Autodesk Inventor part; units mm, degrees
ref_plane "YZ Plane" through (0, 0, 0) normal (1, 0, 0) x (0, 1, 0)
ref_plane "XZ Plane" through (0, 0, 0) normal (0, 1, 0) x (-1, 0, 0)
ref_plane "XY Plane" through (0, 0, 0) normal (0, 0, 1) x (1, 0, 0)
sketch "Sketch1" plane through (0, 0, 0) normal (0, 0, 1) x (1, 0, 0)
  line L0 (-107.95, 63.5) -> (107.95, 63.5)
  line L1 (107.95, 63.5) -> (107.95, -63.5)
  line L2 (107.95, -63.5) -> (-107.95, -63.5)
  line L3 (-107.95, -63.5) -> (-107.95, 63.5)
  line L4 (-107.95, 63.5) -> (107.95, -63.5) construction
  line L5 (107.95, 63.5) -> (-107.95, -63.5) construction
  point P0 (0, 0)
  dimension "d0" = 215.9
  dimension "d1" = 127
extrude "Extrusion1" add sketch "Sketch1" along normal blind 317.5
fillet "Fillet1" radius 10 12 edges at (0, 63.5, 317.5) (-107.95, 63.5, 158.75) (0, 63.5, 0) (107.95, 63.5, 158.75) (107.95, 0, 317.5) (107.95, -63.5, 158.75) (107.95, 0, 0) (0, -63.5, 317.5) (-107.95, 0, 317.5) (0, -63.5, 0) (-107.95, 0, 0) (-107.95, -63.5, 158.75)
sketch "Sketch4" plane through (-97.95, 63.5, 10) normal (0, 1, 0) x (1, 0, 0)
  line L0 (10, -10) -> (185.9, -10)
  line L1 (185.9, -10) -> (185.9, -287.5)
  line L2 (185.9, -287.5) -> (10, -287.5)
  line L3 (10, -287.5) -> (10, -10)
  line L4 (0, 0) -> (195.9, 0)
  line L5 (195.9, 0) -> (195.9, -297.5)
  line L6 (195.9, -297.5) -> (0, -297.5)
  line L7 (0, -297.5) -> (0, 0)
  point P0 (97.95, 10)
  point P1 (97.95, -10)
  dimension "d20" = 10
  dimension "d21" = 10
  dimension "d22" = 10
  dimension "d23" = 10
extrude "Extrusion4" cut sketch "Sketch4" against normal blind 110 contours L0 L1 L2 L3
sketch "Sketch5" plane through (107.95, -53.5, 10) normal (1, 0, 0) x (0, 0, -1)
  circle A0 centre (-267.75, 94.1117) radius 10
  circle A1 centre (-208.25, 94.1117) radius 10
  circle A2 centre (-148.75, 94.1117) radius 10
  circle A3 centre (-89.25, 94.1117) radius 10
  circle A4 centre (-29.75, 94.1117) radius 10
  line L0 (-297.5, 107) -> (-297.5, 0)
  point P0 (10, 53.5)
  dimension "d26" = 20
  dimension "d27" = 20
  dimension "d28" = 20
  dimension "d29" = 20
  dimension "d30" = 20
  dimension "d31" = 29.75
  dimension "d32" = 59.5
  dimension "d33" = 59.5
  dimension "d34" = 59.5
  dimension "d35" = 59.5
extrude "Extrusion5" cut sketch "Sketch5" against normal blind 59.5
equation "\"d36\" = d33"
Part model, mm, in its own coordinate system. A direction names the side the tool comes from. Coordinates: 2 decimals unless noted, no trailing zeros. Loops run counter-clockwise (first coordinate to the right, second up) from the corner with the lowest first, then second, coordinate; pieces in that order, holes last. Notation, with made-up numbers: (-14, 16.25) - (42, 16.25) arc R24 ccw to (42, 45.25) - close; hole circle Ø4 at (-5, -36). An arc over 180 degrees is marked (long way). Write item = value, one per line. Start each with the question number.
Item 1: Cut at B-B, the plane y = 23. Give the cut face in (x, z).
Item 2: Cut at A-A, the plane z = 277.75. Give the cut face in (x, y).
Item 3: Cut at D-D, the plane z = 200.5. Give the cut face in (x, y), and give its area (3 significant figures).
Item 4: Flat gauge pins, fed straight in: pin 1 Ø3 at (x, y) = (-27.5, 35) entering from -Z; pin 2 Ø2 at (x, z) = (-69, 129.5) entering from +Y. Where does each tip first touch, or does it go through?
Item 5: Mould opens along Z. For faces 1 (the cylindrical face through (98.09, 36.782, 209.013)), 2 (the cylindrical face through (104.94, -0.75, 2.85)), 3 (the cylindrical face through (105.1, -0.75, 314.49)), 4 (the cylindrical face through (105.1, 60.49, 160.83)) say: released by +Z, released by -Z, zero draft, split by the parting line, or undercut.
Item 6: Wall check: L1, parallel to Y at x = 97, z = 158.75; L2, parallel to X at y = 16.5, z = 152; L3, parallel to Z at x = 34.5, y = 14.5. Give the ranges that are in metal, low to high. Write a range as from..to.
Item 7: Cut at C-C, the plane x = 93.5. Give the cut face in (y, z), and give its area (3 significant figures).
Item 8: 3-axis set-ups, long thin cutter, end or side, ignore diameter. For faces 5 (the cylindrical face through (104.94, -60.65, 160.83)), 6 (the cylindrical face through (98.09, 30.85, 41.92)), 7 (the flat face through (-87.95, 9, 161)): which of +Z, -Z, +X, -X, +Y, -Y reach the whole face in a straight line?
The answers:
q1.outline = (-107.95, 10) arc R10 ccw to (-97.95, 0) - (97.95, 0) arc R10 ccw to (107.95, 10) - (107.95, 307.5) arc R10 ccw to (97.95, 317.5) - (-97.95, 317.5) arc R10 ccw to (-107.95, 307.5) - close; hole (-87.95, 20) - (87.95, 20) - (87.95, 297.5) - (-87.95, 297.5) - close
q2.outline = (-107.95, -53.5) arc R10 ccw to (-97.95, -63.5) - (97.95, -63.5) arc R10 ccw to (107.95, -53.5) - (107.95, 30.61) - (87.95, 30.61) - (87.95, -46.5) - (-87.95, -46.5) - (-87.95, 63.5) - (-97.95, 63.5) arc R10 ccw to (-107.95, 53.5) - close; (87.95, 50.61) - (107.95, 50.61) - (107.95, 53.5) arc R10 ccw to (97.95, 63.5) - (87.95, 63.5) - close
q3.outline = (-107.95, -53.5) arc R10 ccw to (-97.95, -63.5) - (97.95, -63.5) arc R10 ccw to (107.95, -53.5) - (107.95, 53.5) arc R10 ccw to (97.95, 63.5) - (87.95, 63.5) - (87.95, -46.5) - (-87.95, -46.5) - (-87.95, 63.5) - (-97.95, 63.5) arc R10 ccw to (-107.95, 53.5) - close
q3.area = 7,980 mm2
q4.pin_1 = 0
q4.pin_2 = -46.5
q5.face_1 = undercut
q5.face_2 = released by -Z
q5.face_3 = released by +Z
q5.face_4 = zero draft
q6.L1 = -63.5..30.61, 50.61..63.5
q6.L2 = -107.95..-87.95, 87.95..107.95
q6.L3 = 0..20, 297.5..317.5
q7.outline = (-63.5, 10) arc R10 ccw to (-53.5, 0) - (53.5, 0) arc R10 ccw to (63.5, 10) - (63.5, 307.5) arc R10 ccw to (53.5, 317.5) - (-53.5, 317.5) arc R10 ccw to (-63.5, 307.5) - close; hole circle Ø20 at (40.61, 39.75); hole circle Ø20 at (40.61, 99.25); hole circle Ø20 at (40.61, 158.75); hole circle Ø20 at (40.61, 218.25); hole circle Ø20 at (40.61, 277.75)
q7.area = 38,700 mm2
q8.face_5 = +Z, -Z, +X, -Y
q8.face_6 = +X
q8.face_7 = +Y
